Can you work these out from the model? Positions are in its coordinate system, mm. A direction names the side the tool comes from. Coordinates: 2 decimals unless noted, no trailing zeros. Loops run counter-clockwise (first coordinate to the right, second up) from the corner with the lowest first, then second, coordinate; pieces in that order, holes last. Notation, with made-up numbers: (84.25, -1) -> (111.25, -1) arc R27 cw to (111.25, 34) -> close; hole circle Ø7 at (37, 19.5). An arc over 180 degrees is marked (long way). Use one line per item in the form item = value. Start each with the question number.
(1) Imagine slicing it at A-A (x = 53). List the corners of the cut face in (y, z) for me.
(2) Imagine slicing it at D-D (x = 14). List the corners of the cut face in (y, z) for me.
(3) On a 3-axis mill with a long thin cutter (end or side, diameter ignored), from which of +Z, -Z, +X, -X, +Y, -Y can I reach the whole of each face in a straight line? I mean faces 4 (the flat face through (25, 18.034, 6)), 5 (the cylindrical face through (29.827, 0.084, 8.253)), 6 (the flat face through (31.115, 0, 6)). Say none if no direction works.
(4) Thinking about a two-plate mould opening in Z: for faces 1 (the flat face through (40, 0, 0)), 2 (the cylindrical face through (18.03, -0.4, 6.44)), 3 (the flat face through (48, 0, 3.81)), which applies, released by +Z, released by -Z, zero draft, split by the parting line, or undercut?
(5) Imagine slicing it at B-B (y = 0). List the corners of the cut face in (x, z) for me (3 decimals), plus the area to 3 significant figures.
(6) I need wall thicknesses on line 1 (Z direction, x = 39, y = 11); line 2 (Y direction, x = 12.5, z = 8); line 3 (Y direction, x = 6, z = 11). Which ranges of each line are inside material? Lowest first, please. Write a range as [from, to].
(7) Imagine slicing it at C-C (z = 6.35). List the corners of the cut face in (x, y) for me (3 decimals).
(8) I'm going to push a flat-ended pin straight in: pin 1 (2 mm diameter, centred on x = 48.5, z = 6.5, fed in from -Y). Where does the tip first touch, or does it pass through?
```python
from build123d import *

# Parameters (mm, degrees)
SKETCH1_R                = 19.939
CIRCLE_EXTRUDE_DEPTH     = 12.7
SKETCH3_W                = 12.7
SKETCH3_H                = 39.878
RECTANGLE_EXTRUDE_DEPTH  = 68.58
SKETCH2_R                = 18.034
CRICLE_CUT_DEPTH         = 73.54012766
SKETCH4_OUTSIDE_W        = 110.101
SKETCH4_OUTSIDE_H        = 61.46
SKETCH4_OUTSIDE_W_2      = 66.675
SKETCH4_OUTSIDE_H_2      = 36.068
FRAME_CUT_DEPTH          = 73.54012766
SKETCH13_W               = 5.08
SKETCH13_H               = 36.068
BACK_CUT_DEPTH           = 38.1
SKETCH14_R               = 1.905
FOR_SPRING_EXTRUDE_DEPTH = 2.54


with BuildPart() as part:
    # Sketch1 → circle extrude (new body)
    with BuildSketch(Plane.XY):
        Circle(SKETCH1_R)
    extrude(amount=CIRCLE_EXTRUDE_DEPTH)

    # Sketch3 → rectangle extrude (add)
    with BuildSketch(Plane(origin=(0, 0, 0), x_dir=(0, 0, -1), z_dir=(1, 0, 0))):
        with Locations((-6.35, 0)):
            Rectangle(SKETCH3_W, SKETCH3_H)
    extrude(amount=RECTANGLE_EXTRUDE_DEPTH)

    # Sketch2 → cricle cut (cut, through all)
    with BuildSketch(Plane.XY.offset(12.7)):
        Circle(SKETCH2_R)
    extrude(amount=-CRICLE_CUT_DEPTH, mode=Mode.SUBTRACT)

    # Sketch4 outside → frame cut (cut, through all)
    with BuildSketch(Plane.XY.offset(12.7)):
        with Locations((24.3205, 0)):
            Rectangle(SKETCH4_OUTSIDE_W, SKETCH4_OUTSIDE_H)
        with Locations((33.3375, 0)):
            Rectangle(SKETCH4_OUTSIDE_W_2, SKETCH4_OUTSIDE_H_2, mode=Mode.SUBTRACT)
    extrude(amount=-FRAME_CUT_DEPTH, mode=Mode.SUBTRACT)

    # Sketch13 → back cut (cut)
    with BuildSketch(Plane(origin=(66.675, 0, 0), x_dir=(0, 0, -1), z_dir=(1, 0, 0))):
        with Locations((-6.35, 0)):
            Rectangle(SKETCH13_W, SKETCH13_H)
    extrude(amount=-BACK_CUT_DEPTH, mode=Mode.SUBTRACT)

    # Sketch14 → for spring extrude (add)
    with BuildSketch(Plane(origin=(28.575, 0, 0), x_dir=(0, 0, -1), z_dir=(1, 0, 0))):
        with Locations((-6.35, 0)):
            Circle(SKETCH14_R)
    extrude(amount=FOR_SPRING_EXTRUDE_DEPTH)


solid = part.part
```
Worked out:
q1.outline = (-18.03, 0) -> (18.03, 0) -> (18.03, 3.81) -> (-18.03, 3.81) -> close; (-18.03, 8.89) -> (18.03, 8.89) -> (18.03, 12.7) -> (-18.03, 12.7) -> close
q2.outline = (-18.03, 0) -> (-11.37, 0) -> (-11.37, 12.7) -> (-18.03, 12.7) -> close; (11.37, 0) -> (18.03, 0) -> (18.03, 12.7) -> (11.37, 12.7) -> close
q3.face_4 = +Z, -Z, +X, -X, +Y
q3.face_5 = +X
q3.face_6 = +X, +Y, -Y
q4.face_1 = released by -Z
q4.face_2 = zero draft
q4.face_3 = undercut
q5.outline = (18.034, 0) -> (66.675, 0) -> (66.675, 3.81) -> (28.575, 3.81) -> (28.575, 4.445) -> (31.115, 4.445) -> (31.115, 8.255) -> (28.575, 8.255) -> (28.575, 8.89) -> (66.675, 8.89) -> (66.675, 12.7) -> (18.034, 12.7) -> close
q5.area = 434 mm2
q6.line_1 = [0, 3.81], [8.89, 12.7]
q6.line_2 = [-18.03, -13], [13, 18.03]
q6.line_3 = [-18.03, -17.01], [17.01, 18.03]
q7.outline = (0, -18.034) -> (28.575, -18.034) -> (28.575, -1.905) -> (31.115, -1.905) -> (31.115, 1.905) -> (28.575, 1.905) -> (28.575, 18.034) -> (0, 18.034) arc R18.034 cw to start
q8.pin_1 = through
